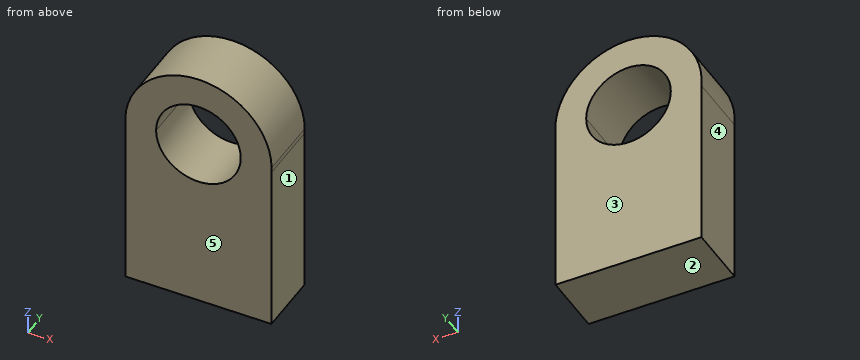
```python
from build123d import *

# Parameters (mm, degrees)
F1_DEPTH = 25.4


with BuildPart() as f1:
    # F0 (on Front) → F1 (new body)
    with BuildSketch(Plane.XZ):
        with BuildLine():
            ThreePointArc((-29.36328, 33.386896), (0, 6.035167), (29.36328, 33.386896))
            Line((29.36328, 33.386896), (29.36328, 35.472415))
            Line((29.36328, 35.472415), (17.021102, 35.472415))
            ThreePointArc((17.021102, 35.472415), (0, 18.451314), (-17.021102, 35.472415))
            Line((-17.021102, 35.472415), (-29.36328, 35.472415))
            Line((-29.36328, 35.472415), (-29.36328, 33.386896))
        make_face()
        with BuildLine():
            Line((-29.36328, -35.472415), (29.36328, -35.472415))
            Line((29.36328, -35.472415), (29.36328, 33.386896))
            ThreePointArc((29.36328, 33.386896), (0, 6.035167), (-29.36328, 33.386896))
            Line((-29.36328, 33.386896), (-29.36328, -35.472415))
        make_face()
        with BuildLine():
            Line((29.36328, 35.472415), (29.36328, 33.386896))
            ThreePointArc((29.36328, 33.386896), (29.418751, 34.429), (29.437249, 35.472415))
            ThreePointArc((29.437249, 35.472415), (-1.043415, 64.891166), (-29.36328, 33.386896))
            Line((-29.36328, 33.386896), (-29.36328, 35.472415))
            Line((-29.36328, 35.472415), (-17.021102, 35.472415))
            ThreePointArc((-17.021102, 35.472415), (0, 52.493517), (17.021102, 35.472415))
            Line((17.021102, 35.472415), (29.36328, 35.472415))
        make_face()
    extrude(amount=F1_DEPTH)


solid = f1.part
```
Check sheet for the modelled part. Datum: model origin and axes. Units: mm. Face numbers are marked on the shaded views. A direction names the side the tool comes from. Round coordinates to 2 decimals unless told otherwise and drop trailing zeros. Order: outer loops, then holes, each group sorted by start corner. A loop starts at its lowest first (then second) coordinate and runs counter-clockwise, first axis right, second up.
1) Tool access check on the marked faces 1 and 2. Record the directions out of +Z, -Z, +X, -X, +Y, -Y that give a thin tool (end or side, any length) a straight path to the whole face; none if there is none.
2) Section check C-C (z = 48). Record the boundary of the cut face in (x, y), and give its area (3 significant figures).
3) Section check A-A (x = 0). Record the boundary of the cut face in (y, z), and give its area (3 significant figures).
4) Mould release check, pull along Y, two halves, no side actions. Record for the marked faces 3, 4 and 5: +Y half, -Y half, draft (parallel to the pull), parting line (faces both ways), or undercut.
5) Section check B-B (y = -9.75). Record the boundary of the cut face in (x, z), and give its area (3 significant figures).
6) Scan lines: line 1 (X direction, y = -23.5, z = -20); line 2 (X direction, y = -21.75, z = 30); line 3 (Z direction, x = -10.5, y = -5.75). Record each from-to range of solid material in increasing order.
7) Go/stop test with flat-tipped pins: pin 1 Ø3 at (x, z) = (21.5, 23) entering from +Y; pin 2 Ø6 at (x, y) = (9, -12) entering from +Z; pin 3 Ø5 at (y, z) = (-13.5, 31.5) entering from -X; pin 4 Ø7.5 at (y, z) = (-13, 10.5) entering from +X. Record where each tip stops, or that it passes through.
Result:
1. face 1: -Z, +X, +Y, -Y
1. face 2: -Z, +X, -X, +Y, -Y
2. outline: (-26.64, -25.4) - (-11.52, -25.4) - (-11.52, 0) - (-26.64, 0) - close; (11.52, -25.4) - (26.64, -25.4) - (26.64, 0) - (11.52, 0) - close
2. area: 768 mm2
3. outline: (-25.4, -35.47) - (0, -35.47) - (0, 18.45) - (-25.4, 18.45) - close; (-25.4, 52.49) - (0, 52.49) - (0, 64.91) - (-25.4, 64.91) - close
3. area: 1,690 mm2
4. face 3: +Y half
4. face 4: draft
4. face 5: -Y half
5. outline: (-29.36, -35.47) - (29.36, -35.47) - (29.36, 33.39) arc R29.44 ccw to (29.44, 35.47) arc R29.44 ccw (long way) to (-29.36, 33.39) - close; hole (-17.02, 35.47) arc R17.02 ccw to (17.02, 35.47) arc R17.02 ccw to start
5. area: 4,620 mm2
6. line 1: x = -29.36 to 29.36
6. line 2: x = -29.36 to -16.12, 16.12 to 29.36
6. line 3: z = -35.47 to 22.08, 48.87 to 62.97
7. pin 1: stops at y = 0
7. pin 2: stops at z = 64.29
7. pin 3: stops at x = -29.4
7. pin 4: stops at x = 29.36
